Input: dimensioned drawing with shaded views. Units: mm. Origin: part minimum x, y, z. A direction names the side the tool comes from. Give positions to 0.01 mm unless a question says otherwise; leave off trailing zeros. Loops run counter-clockwise (first coordinate to the right, second up) from the corner with the lowest first, then second, coordinate; pieces in that order, holes last. Notation, with made-up numbers: (72.5, -5.5) -> (110.5, -5.5) arc R10 cw to (110.5, 4.5) -> close; hole circle Ø1 at (-16, 46). An arc over 180 degrees is marked (long way). Answer in a Markdown table with one row per item. Add a question column.
1) Section query B-B (z = 93). Return the cut outline in (x, y).
2) Section query A-A (x = 185.5). Return the cut outline in (y, z).
3) First-contact query: P1, Ø4, axis at y = 282, z = 74, coming from the -X side; P2, Ø3, axis at x = 168.5, z = 50.5, coming from the -Y side (1 decimal); P3, Ø1.5, axis at y = 198.5, z = 144.5, coming from the -X side (1 decimal). Flat tips, straight axial feed; report the tip coordinate or a pass-through.
4) Line query: line 1 (Z direction, x = 205, y = 45.5); line 2 (X direction, y = 291.5, z = 44.5) (1 decimal); line 3 (Y direction, x = 179, z = 96.5) (1 decimal). Output: solid intervals per line, ascending. Write a range as from..to.
5) Section query C-C (y = 164). Return the cut outline in (x, z).
6) Access query for the marked faces 1 and 2. Directions: +Z, -Z, +X, -X, +Y, -Y. A direction counts if a zero-diameter tool reaches every point of the face in a straight line with its end or side. Return the directions, or none.
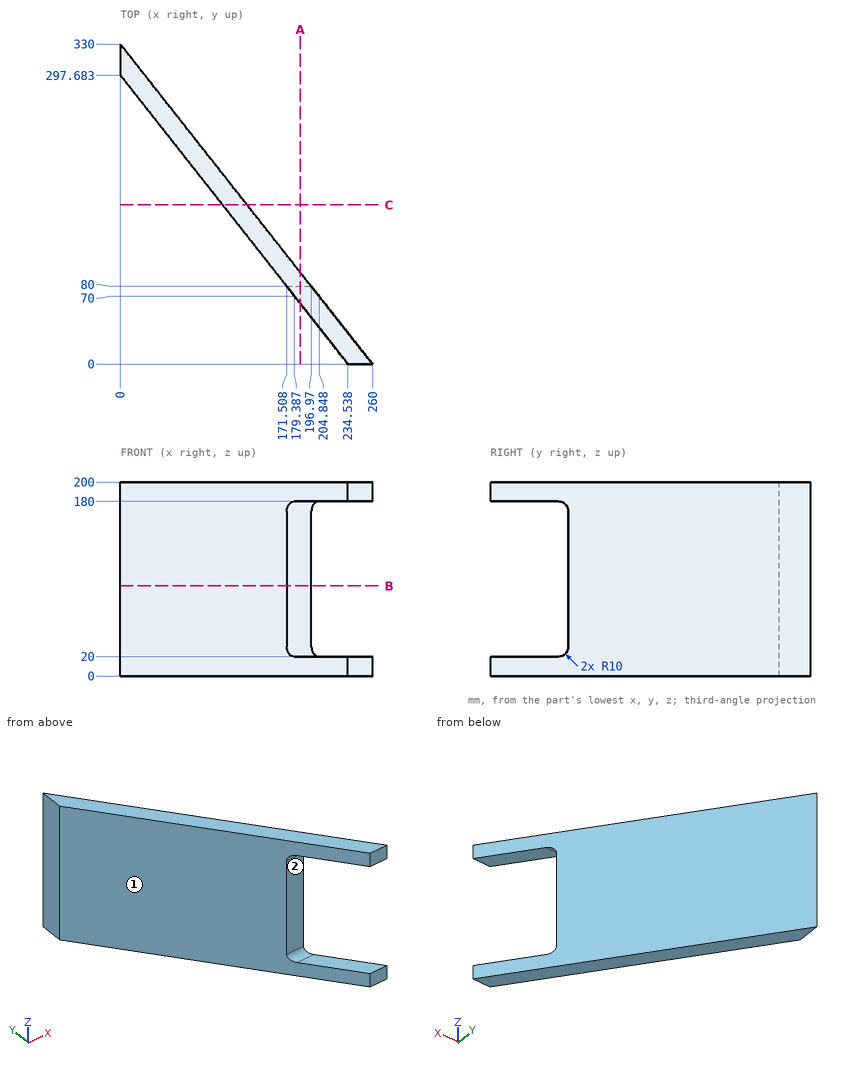
Evaluation:
| question | item | result |
|---|---|---|
| 1 | outline | (0, 297.68) -> (171.51, 80) -> (196.97, 80) -> (0, 330) -> close |
| 2 | outline | (62.24, 0) -> (94.56, 0) -> (94.56, 200) -> (62.24, 200) -> (62.24, 180) -> (70, 180) arc R10 cw to (80, 170) -> (80, 30) arc R10 cw to (70, 20) -> (62.24, 20) -> close |
| 3 | P1 | x = 10.78 |
| 3 | P2 | y = 81.9 |
| 3 | P3 | x = 77.6 |
| 4 | line 1 | 0..20, 180..200 |
| 4 | line 2 | 4.9..30.3 |
| 4 | line 3 | 80..102.8 |
| 5 | outline | (105.33, 0) -> (130.79, 0) -> (130.79, 200) -> (105.33, 200) -> close |
| 6 | face 1 | +Z, -Z, -X, -Y |
| 6 | face 2 | +X, -X, -Y |
